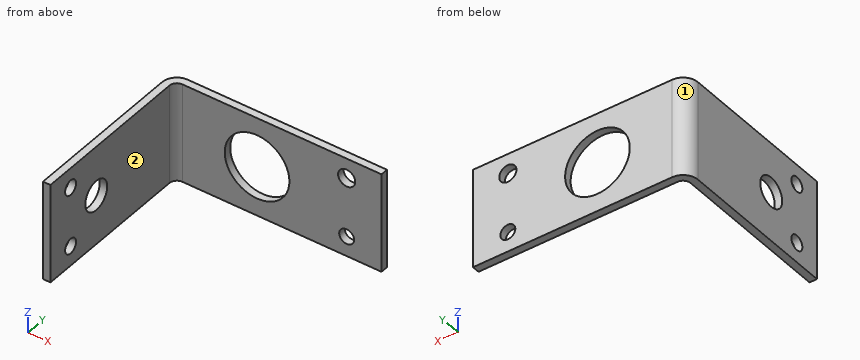
```python
from build123d import *

# Parameters (mm, degrees)
BASE_FLANGE1_DEPTH = 40
SKETCH2_R          = 6
CUT_EXTRUDE1_DEPTH = 115.512008104
SKETCH3_R          = 13
CUT_EXTRUDE2_DEPTH = 117.704755687
SKETCH4_R          = 3
CUT_EXTRUDE3_DEPTH = 10
SKETCH5_R          = 3
SKETCH5_R_2        = 3.446989576
CUT_EXTRUDE4_DEPTH = 10


# Sheet-metal steps are written as plain solids
with BuildPart() as part:
    # Sketch1 → Base-Flange1 (new body)
    with BuildSketch(Plane.XY):
        with BuildLine():
            Line((0, 0), (-80, 0))
            ThreePointArc((-80, 0), (-82.121320344, -0.878679656), (-83, -3))
            Line((-83, -3), (-83, -68))
            Line((-83, -68), (-86, -68))
            Line((-86, -68), (-86, -3))
            ThreePointArc((-86, -3), (-84.242640687, 1.242640687), (-80, 3))
            Line((-80, 3), (0, 3))
            Line((0, 3), (0, 0))
        make_face()
    extrude(amount=BASE_FLANGE1_DEPTH)

    # Sketch2 → Cut-Extrude1 (cut, through all)
    with BuildSketch(Plane(origin=(-83, 0, 0), x_dir=(0, 0, -1), z_dir=(1, 0, 0))):
        with Locations(Location((-20, -43, 0), (0, 0, 90))):
            Circle(SKETCH2_R)
    extrude(amount=-CUT_EXTRUDE1_DEPTH, mode=Mode.SUBTRACT)

    # Sketch3 → Cut-Extrude2 (cut, through all)
    with BuildSketch(Plane.XZ):
        with Locations((-50.000101558, 20)):
            Circle(SKETCH3_R)
    extrude(amount=-CUT_EXTRUDE2_DEPTH, mode=Mode.SUBTRACT)

    # Sketch4 → Cut-Extrude3 (cut)
    with BuildSketch(Plane(origin=(-83, 0, 0), x_dir=(0, 0, -1), z_dir=(1, 0, 0))):
        with Locations(Location((-8, -57, 0), (0, 0, 90))):
            Circle(SKETCH4_R)
        with Locations(Location((-32, -57, 0), (0, 0, 90))):
            Circle(SKETCH4_R)
    extrude(amount=-CUT_EXTRUDE3_DEPTH, mode=Mode.SUBTRACT)

    # Sketch5 → Cut-Extrude4 (cut)
    with BuildSketch(Plane.XZ):
        with Locations((-14, 8)):
            Circle(SKETCH5_R)
        with Locations((-14, 32)):
            Circle(SKETCH5_R_2)
    extrude(amount=-CUT_EXTRUDE4_DEPTH, mode=Mode.SUBTRACT)


solid = part.part
```
Input: part model. Units: mm. Frame: model coordinates. Face numbers are marked on the shaded views. A direction names the side the tool comes from. Give positions to 0.01 mm unless a question says otherwise; leave off trailing zeros. Order: outer loops, then holes, each group sorted by start corner. A loop starts at its lowest first (then second) coordinate and runs counter-clockwise, first axis right, second up. Notation, with made-up numbers: M 83,35.5 L 138,35.5 A11 ccw 138,43.5 Z; hole C -12.75,53.25 d8. An arc over 180 degrees is marked long. One line per question, with ' | ' between items. Start each with the question number.
1. Material intervals for probe 1 along Z at (x, y) = (-85.2, -57); probe 2 along Z at (x, y) = (-14, 2.45); probe 3 along Z at (x, y) = (-85, -43), sorted ascending. Write a range as [from, to].
2. First-contact query: pin 1 Ø20 at (y, z) = (-34, 28) entering from +X; pin 2 Ø11 at (x, z) = (-14, 32) entering from -Y; pin 3 Ø23.5 at (x, z) = (-50, 20) entering from +Y. Flat tips, straight axial feed; report the tip coordinate or a pass-through.
3. Section query C-C (y = -57). Return the cut outline in (x, z), and give its area (3 significant figures).
4. Section query A-A (x = -14). Return the cut outline in (y, z), and give its area (3 significant figures).
5. Section query D-D (y = -38). Return the cut outline in (x, z), and give its area (3 significant figures).
6. Section query B-B (z = 20). Return the cut outline in (x, y).
7. Access query for the marked faces 1 and 2. Directions: +Z, -Z, +X, -X, +Y, -Y. A direction counts if a zero-diameter tool reaches every point of the face in a straight line with its end or side. Return the directions, or none.
Here are the results:
1) probe 1: [0, 5], [11, 29], [35, 40] | probe 2: [0, 5], [11, 28.55], [35.45, 40] | probe 3: [0, 14], [26, 40]
2) pin 1: x = -83 | pin 2: y = 0 | pin 3: through
3) outline: M -86,0 L -83,0 L -83,5 L -86,5 Z; M -86,11 L -83,11 L -83,29 L -86,29 Z; M -86,35 L -83,35 L -83,40 L -86,40 Z | area: 84.0 mm²
4) outline: M 0,0 L 3,0 L 3,5 L 0,5 Z; M 0,11 L 3,11 L 3,28.55 L 0,28.55 Z; M 0,35.45 L 3,35.45 L 3,40 L 0,40 Z | area: 81.3 mm²
5) outline: M -86,0 L -83,0 L -83,16.68 L -86,16.68 Z; M -86,23.32 L -83,23.32 L -83,40 L -86,40 Z | area: 100 mm²
6) outline: M -86,-68 L -83,-68 L -83,-49 L -86,-49 Z; M -86,-37 L -83,-37 L -83,-3 A3 cw -80,0 L -63,0 L -63,3 L -80,3 A6 ccw -86,-3 Z; M -37,0 L 0,0 L 0,3 L -37,3 Z
7) face 1: +Z, -Z, -X, +Y | face 2: +Z, -Z, +X, -Y
